Geometry: final body of the model. Coordinates: model frame, mm. A direction names the side the tool comes from. Round coordinates to 2 decimals unless told otherwise and drop trailing zeros. Loops run counter-clockwise (first coordinate to the right, second up) from the corner with the lowest first, then second, coordinate; pieces in that order, holes last. Notation, with made-up numbers: (32, 86.25) -> (56, 86.25) arc R31 ccw to (56, 118.25) -> close; hole circle Ø4 at (7, 68.25). An arc over 180 degrees is marked (long way). Answer in a Markdown table with one row per item.
```python
from build123d import *

# Parameters (mm, degrees)
SKETCH1_R                = 3.175
BOSS_EXTRUDE1_DEPTH      = 38.1
BOSS_EXTRUDE2_DEPTH      = 6.35
FILLET1_R                = 3.175
BOSS_EXTRUDE3_DEPTH      = 3.81
BOSS_EXTRUDE3_DEPTH_BACK = 10.16
SKETCH3_W                = 12.7
SKETCH3_H                = 63.5
FILLET2_R                = 3.175
FILLET3_R                = 6.35
CUT_EXTRUDE1_REACH       = 94.13
SKETCH4_W                = 15.24
SKETCH4_H                = 7.62
SKETCH5_R                = 3.175
BOSS_EXTRUDE4_DEPTH      = 10.16
BOSS_EXTRUDE5_START      = 38.1
SKETCH6_R                = 3.175
BOSS_EXTRUDE5_DEPTH      = 38.1
SKETCH7_R                = 3.175
CUT_EXTRUDE2_DEPTH       = 38.1


with BuildPart() as part:
    # Sketch1 → Boss-Extrude1 (new body)
    with BuildSketch(Plane(origin=(0, 0, 0), x_dir=(1, 0, 0), z_dir=(0, 1, 0))):
        with Locations(Location((0, 0, 0), (0, 0, 270))):
            Circle(SKETCH1_R)
    extrude(amount=-BOSS_EXTRUDE1_DEPTH)

    # Sketch2 → Boss-Extrude2 (add)
    with BuildSketch(Plane(origin=(0, 0, 0), x_dir=(1, 0, 0), z_dir=(0, 1, 0))):
        Polygon((34.925, -3.175), (-3.175, -3.175), (-3.175, 3.175), (28.575, 3.175), (28.575, 60.325), (34.925, 60.325), align=None)
    extrude(amount=BOSS_EXTRUDE2_DEPTH)

    # Fillet1
    fillet1_edges = [part.edges().sort_by_distance(p)[0] for p in [
        (28.575, 3.175, -3.175),
        (34.925, 3.175, 3.175),
        (-3.175, 3.175, -3.175),
        (-3.175, 3.175, 3.175),
    ]]
    fillet(fillet1_edges, radius=FILLET1_R - 0.0001)  # a hair under: the kernel refuses the full size

    # Sketch3 → Boss-Extrude3 (add, two sides: drawn at the far end of the back side and taken through both)
    with BuildSketch(Plane(origin=(0, 6.35, 0), x_dir=(1, 0, 0), z_dir=(0, 1, 0)).offset(-BOSS_EXTRUDE3_DEPTH_BACK)):
        with Locations((31.75, 41.275)):
            Rectangle(SKETCH3_W, SKETCH3_H)
    extrude(amount=BOSS_EXTRUDE3_DEPTH + BOSS_EXTRUDE3_DEPTH_BACK)

    # Fillet2
    fillet2_edges = [part.edges().sort_by_distance(p)[0] for p in [
        (28.575, 3.175, -9.525),
        (31.75, 0, -9.525),
        (34.925, 3.175, -9.525),
        (31.75, 6.35, -9.525),
    ]]
    fillet(fillet2_edges, radius=FILLET2_R - 0.0001)  # a hair under: the kernel refuses the full size

    # Fillet3
    fillet3_edges = [part.edges().sort_by_distance(p)[0] for p in [
        (25.4, 3.175, -73.025),
        (38.1, 3.175, -73.025),
    ]]
    fillet(fillet3_edges, radius=FILLET3_R - 0.0001)  # a hair under: the kernel refuses the full size

    # Sketch4 → Cut-Extrude1 (cut, up to next)
    with BuildSketch(Plane(origin=(38.1, 0, 0), x_dir=(0, 0, -1), z_dir=(1, 0, 0)), mode=Mode.PRIVATE) as cut_extrude1_sk1:
        with Locations((66.675, 3.175)):
            Rectangle(SKETCH4_W, SKETCH4_H)
    cut_extrude1_tool1 = extrude(cut_extrude1_sk1.sketch, amount=-CUT_EXTRUDE1_REACH, mode=Mode.PRIVATE) & part.part
    add(cut_extrude1_tool1.solids().sort_by_distance((38.1, 3.175, -66.675))[0], mode=Mode.SUBTRACT)

    # Sketch5 → Boss-Extrude4 (add)
    with BuildSketch(Plane(origin=(0, -0.635, 0), x_dir=(1, 0, 0), z_dir=(0, 1, 0))):
        with Locations(Location((31.75, 66.675, 0), (0, 0, 90))):
            Circle(SKETCH5_R)
    extrude(amount=BOSS_EXTRUDE4_DEPTH)

    # Sketch6 → Boss-Extrude5 (add)
    with BuildSketch(Plane(origin=(0, 6.35, 0), x_dir=(1, 0, 0), z_dir=(0, 1, 0)).offset(BOSS_EXTRUDE5_START)):
        with Locations(Location((0, 0, 0), (0, 0, 270))):
            Circle(SKETCH6_R)
    extrude(amount=-BOSS_EXTRUDE5_DEPTH)

    # Sketch7 → Cut-Extrude2 (cut)
    with BuildSketch(Plane.XZ):
        with Locations(Location((0, 0, 0), (0, 0, 90))):
            Circle(SKETCH7_R)
    extrude(amount=CUT_EXTRUDE2_DEPTH, mode=Mode.SUBTRACT)


with BuildPart() as cut_extrude2_kept_piece:
    # of the separate pieces the step leaves, the one the design keeps (cut_extrude2_pieces_kept)
    add(part.part.solids().sort_by_distance((25.4, 10.16, -66.6751))[0])


solid = cut_extrude2_kept_piece.part
```
Item 1: Mould query, pull axis Z, two halves, no side actions, for faces 1 (the cylindrical face through (31.84, -1.38, -8.97)), 2 (the cylindrical face through (34.85, 3.12, -65.99)), 3 (the flat face through (32, 3, -59.055)), 4 (the flat face through (0, 44.45, 0)). Classes: released by +Z, released by -Z, zero draft, split by the parting line, or undercut.
Ans:
| item | result |
|---|---|
| face 1 | released by +Z |
| face 2 | undercut |
| face 3 | undercut |
| face 4 | zero draft |
Item 2: Section query C-C, the plane x = 4. Output: boundary loops of the cut face in (y, z) (3 decimals).
Ans:
| item | result |
|---|---|
| outline | (0, -3.175) -> (6.35, -3.175) -> (6.35, 3.175) -> (0, 3.175) -> close |
Item 3: Set-up query: faces 5 (the flat face through (34.925, 3, -3)), 6 (the cylindrical face through (-1.93, 25.67, -2.52)), 7 (the flat face through (25.4, 3, -38)), 8 (the flat face through (32, 6.985, -63)), 9 (the cylindrical face through (36.289, 8.595, -71.116)). Return all of +Z, -Z, +X, -X, +Y, -Y with unobstructed straight access to the full face (end or side cutting, diameter ignored); none if empty.
Ans:
| item | result |
|---|---|
| face 5 | +Z, +X, +Y, -Y |
| face 6 | +Y |
| face 7 | -Z, -X, +Y, -Y |
| face 8 | none |
| face 9 | -Z, +X, +Y, -Y |
Item 4: Ray query, L1, parallel to Y at x = 33, z = -70 (3 decimals); L2, parallel to Y at x = 30, z = -47.5; L3, parallel to Z at x = 21.5, y = 2.5 (3 decimals). Return the intervals inside material, ascending.
Ans:
| item | result |
|---|---|
| L1 | -3.81 to -0.635, 6.985 to 10.16 |
| L2 | -3.81 to 10.16 |
| L3 | -3.175 to 3.175 |
Item 5: Section query D-D, the plane z = -13.5. Output: boundary loops of the cut face in (x, y), and give its area (3 significant figures).
Ans:
| item | result |
|---|---|
| outline | (25.4, -3.81) -> (38.1, -3.81) -> (38.1, 10.16) -> (25.4, 10.16) -> close |
| area | 177 mm2 |
Item 6: First-contact query: P1, Ø6.5, axis at x = 31, z = -55, coming from the +Y side; P2, Ø6, axis at x = 7.5, y = 16.5, coming from the -Z side; P3, Ø4, axis at x = 30.5, y = 4.5, coming from the -Z side; P4, Ø7, axis at x = 7, y = 2, coming from the -Z side (3 decimals). Flat tips, straight axial feed; report the tip coordinate or a pass-through.
Ans:
| item | result |
|---|---|
| P1 | y = 10.16 |
| P2 | through |
| P3 | z = -69.85 |
| P4 | z = -3.175 |
Item 7: Section query B-B, the plane x = 27.5. Output: boundary loops of the cut face in (y, z) (3 decimals).
Ans:
| item | result |
|---|---|
| outline | (-3.81, -71.393) -> (-0.635, -71.393) -> (-0.635, -59.055) -> (6.985, -59.055) -> (6.985, -71.393) -> (10.16, -71.393) -> (10.16, -9.525) -> (9.525, -9.525) arc R3.175 cw to (7.425, -8.731) -> (-1.075, -8.731) arc R3.175 cw to (-3.175, -9.525) -> (-3.81, -9.525) -> close; (0, -3.969) -> (6.35, -3.969) -> (6.35, 3.175) -> (0, 3.175) -> close |
